Design review of the part built by this model. Coordinates are the model's own, in mm. Face numbers are marked on the shaded views. A direction names the side the tool comes from. Give positions to 0.01 mm unless a question says otherwise; leave off trailing zeros. Write each loop counter-clockwise with the first axis right and the second up, starting at its lowest first coordinate (ties: lowest second). Pieces come first, ordered by that corner, then holes. Notation, with made-up numbers: (85, -39) -> (140, -39) arc R28 ccw to (140, -14) -> close; hole circle Ø10 at (-12.75, 79.5). An arc over 180 degrees is marked (long way). Answer as a JSON object with one key per item and string values.
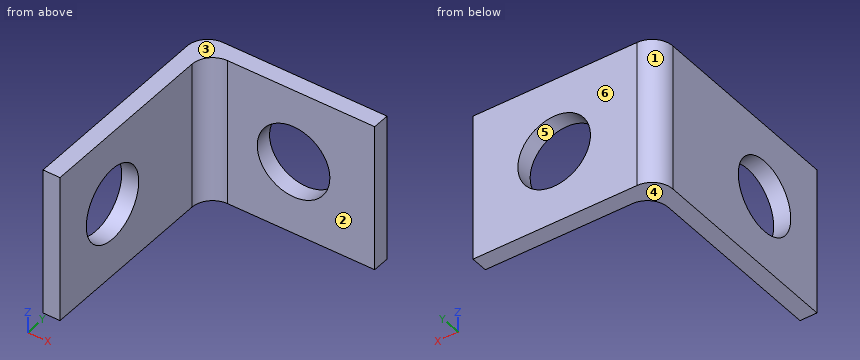
Autodesk Inventor part; units mm, degrees
ref_plane "YZ Plane" through (0, 0, 0) normal (1, 0, 0) x (0, 1, 0)
ref_plane "XZ Plane" through (0, 0, 0) normal (0, 1, 0) x (-1, 0, 0)
ref_plane "XY Plane" through (0, 0, 0) normal (0, 0, 1) x (1, 0, 0)
sketch "Sketch1" plane through (0, 0, 0) normal (0, 0, 1) x (1, 0, 0)
  line L0 (-4.455, 5.305) -> (4.455, 5.305)
  line L1 (4.455, 5.305) -> (4.455, -5.305)
  line L2 (4.455, -5.305) -> (-4.455, -5.305)
  line L3 (-4.455, -5.305) -> (-4.455, 5.305)
  line L4 (-6.237, 0) -> (6.237, 0)
  line L5 (0, -7.427) -> (0, 7.427)
  point P0 (0, 0)
  dimension "d0" = 8.91
  dimension "d1" = 10.61
  dimension "d2" = 4.455
  dimension "d3" = 5.305
extrude "BraketBase" add sketch "Sketch1" along normal blind 7.13
sketch "Sketch2" plane through (0, 0, 7.13) normal (0, 0, 1) x (1, 0, 0)
  line L0 (4.455, 5.305) -> (-4.455, 5.305)
  line L1 (-4.455, 5.305) -> (-4.455, -5.305)
  line L2 (-4.455, -5.305) -> (4.455, -5.305)
  line L3 (4.455, -5.305) -> (4.455, 5.305)
  line L4 (-3.635, 4.485) -> (4.455, 4.485)
  line L5 (-3.635, 4.485) -> (-3.635, -5.305)
  line L6 (-4.455, -5.305) -> (4.455, -5.305)
  line L7 (-3.635, 4.485) -> (4.455, 4.485)
  line L8 (4.455, 4.485) -> (4.455, -5.305)
  line L9 (4.455, -5.305) -> (-3.635, -5.305)
  line L10 (-3.635, -5.305) -> (-3.635, 4.485)
  point P0 (0, 0)
  dimension "d6" = 0.82
  dimension "d7" = 0.82
extrude "BraketCut" cut sketch "Sketch2" against normal blind 7.13 contours L3 L2 L5 L4
sketch "Sketch3" plane through (-4.455, 5.305, 0) normal (0, 1, 0) x (1, 0, 0)
  line L0 (0, 0) -> (8.91, 0)
  line L1 (0, 0) -> (0, -7.13)
  line L2 (8.91, -7.13) -> (0, -7.13)
  line L3 (8.91, 0) -> (8.91, -7.13)
  circle A0 centre (5, -3.565) radius 1.75
  point P0 (4.455, 0)
  dimension "d10" = 3.5
  dimension "d11" = 5
  dimension "d12" = 3.565
hole "ShortHole" at (0.545, 5.305, 3.565) direction (0, -1, 0) diameter 3.5 end through all
sketch "Sketch4" plane through (-3.635, -5.305, 7.13) normal (1, 0, 0) x (0, 0, -1)
  line L0 (0, 0) -> (0, 9.79)
  line L1 (7.13, 0) -> (0, 0)
  line L2 (7.13, 9.79) -> (7.13, 0)
  line L3 (0, 9.79) -> (7.13, 9.79)
  circle A0 centre (3.565, 3.5) radius 1.75
  point P0 (7.13, 5.305)
  dimension "d20" = 3.5
  dimension "d21" = 3.5
  dimension "d22" = 3.565
hole "LongHole" at (-3.635, -1.805, 3.565) direction (-1, 0, 0) diameter 3.5 end through all
fillet "Fillet1" radius 1 2 edges at (-4.455, 5.305, 3.565) (-3.635, 4.485, 3.565)
equation "\"d2\" = 0.5 * d0"
equation "\"d3\" = 0.5 * d1"
equation "\"d7\" = d6"
properties part number "LBracket"
(1) We need section C-C, the plane z = 3. State the section outline as (x, y) points (3 decimals), then the cut area to 3 significant figures.
Here are the results:
{"outline": "(-4.455, -5.305) -> (-3.635, -5.305) -> (-3.635, -3.461) -> (-4.455, -3.461) -> close; (-4.455, -0.149) -> (-3.635, -0.149) -> (-3.635, 3.485) arc R1 cw to (-2.635, 4.485) -> (-1.111, 4.485) -> (-1.111, 5.305) -> (-3.455, 5.305) arc R1 ccw to (-4.455, 4.305) -> close; (2.201, 4.485) -> (4.455, 4.485) -> (4.455, 5.305) -> (2.201, 5.305) -> close", "area": "9.90 mm²"}
(2) The part is to be moulded in two halves that separate along Z. For the marked faces 3, 4, 5 and 6, say which applies: +Z half, -Z half, draft (parallel to the pull), parting line (faces both ways), or undercut.
Here are the results:
{"face 3": "+Z half", "face 4": "-Z half", "face 5": "undercut", "face 6": "draft"}
(3) Clearance check with a flat-ended pin moving along its axis: pin 1 (2 mm diameter, centred on x = -1, z = 4, fed in from -Y) (3 decimals). State where the tip first meets the part, or that it passes through.
Here are the results:
{"pin 1": "stops at y = 4.485"}
(4) For line 1 along X through (y, z) = (-0.5, 6) (3 decimals); line 2 along Z through (x, y) = (1.5, 5); line 3 along Y through (x, z) = (0.5, 1.5) (3 decimals), list the stretches that pass through material, from the lowest coordinate up.
Here are the results:
{"line 1": "x = -4.455 to -3.635", "line 2": "z = 0 to 2.1, 5.03 to 7.13", "line 3": "y = 4.485 to 5.305"}
(5) For the marked faces 1 and 2, list the 3-axis set-ups (+Z, -Z, +X, -X, +Y, -Y) from which the entire face can be reached by the end or side of a thin tool; tool diameter is ignored.
Here are the results:
{"face 1": "+Z, -Z, -X, +Y", "face 2": "+Z, -Z, +X, -Y"}
(6) We need section B-B, the plane x = 1.75. State the section outline as (y, z) points (3 decimals).
Here are the results:
{"outline": "(4.485, 0) -> (5.305, 0) -> (5.305, 2.296) -> (4.485, 2.296) -> close; (4.485, 4.834) -> (5.305, 4.834) -> (5.305, 7.13) -> (4.485, 7.13) -> close"}
(7) We need section D-D, the plane z = 2. State the section outline as (x, y) points (3 decimals).
Here are the results:
{"outline": "(-4.455, -5.305) -> (-3.635, -5.305) -> (-3.635, -2.588) -> (-4.455, -2.588) -> close; (-4.455, -1.022) -> (-3.635, -1.022) -> (-3.635, 3.485) arc R1 cw to (-2.635, 4.485) -> (-0.238, 4.485) -> (-0.238, 5.305) -> (-3.455, 5.305) arc R1 ccw to (-4.455, 4.305) -> close; (1.328, 4.485) -> (4.455, 4.485) -> (4.455, 5.305) -> (1.328, 5.305) -> close"}
(8) We need section A-A, the plane y = -2.5. State the section outline as (x, z) points (3 decimals), then the cut area to 3 significant figures.
Here are the results:
{"outline": "(-4.455, 0) -> (-3.635, 0) -> (-3.635, 1.959) -> (-4.455, 1.959) -> close; (-4.455, 5.171) -> (-3.635, 5.171) -> (-3.635, 7.13) -> (-4.455, 7.13) -> close", "area": "3.21 mm²"}
